Verification items for the finished model (mm, model axes). Face numbers are marked on the shaded views. Round coordinates to 2 decimals unless told otherwise and drop trailing zeros. Loops run counter-clockwise (first coordinate to the right, second up) from the corner with the lowest first, then second, coordinate; pieces in that order, holes last. Notation, with made-up numbers: (48.5, -34) - (78.5, -34) arc R23 ccw to (78.5, -26) - close; hole circle Ø7 at (31.5, 12). An arc over 180 degrees is marked (long way). Use CSV: the item, a comma, the result in double quotes.
```python
from build123d import *

# Parameters (mm, degrees)
SKETCH1_W           = 399
SKETCH1_H           = 246
BOSS_EXTRUDE1_DEPTH = 18
SKETCH2_W           = 239
SKETCH2_H           = 86
CUT_EXTRUDE1_DEPTH  = 6
CUT_EXTRUDE2_REACH  = 290.215


with BuildPart() as part:
    # Sketch1 → Boss-Extrude1 (new body)
    with BuildSketch(Plane(origin=(0, 0, 0), x_dir=(1, 0, 0), z_dir=(0, 1, 0))):
        with Locations((26.513776337, -54.93719611)):
            Rectangle(SKETCH1_W, SKETCH1_H)
    extrude(amount=BOSS_EXTRUDE1_DEPTH)

    # Sketch2 → Cut-Extrude1 (cut)
    with BuildSketch(Plane.XZ):
        with Locations((26.513776337, 54.93719611)):
            Rectangle(SKETCH2_W, SKETCH2_H)
    extrude(amount=-CUT_EXTRUDE1_DEPTH, mode=Mode.SUBTRACT)

    # Sketch3 → Cut-Extrude2 (cut, up to next)
    with BuildSketch(Plane(origin=(0, 18, 0), x_dir=(1, 0, 0), z_dir=(0, 1, 0)), mode=Mode.PRIVATE) as cut_extrude2_sk1:
        Polygon((34.013776337, 68.06280389), (19.013776337, 68.06280389), (11.513776337, 50.06280389), (11.513776337, 30.06280389), (41.513776337, 30.06280389), (41.513776337, 50.06280389), align=None)
    cut_extrude2_tool1 = extrude(cut_extrude2_sk1.sketch, amount=-CUT_EXTRUDE2_REACH, mode=Mode.PRIVATE) & part.part
    add(cut_extrude2_tool1.solids().sort_by_distance((26.513776, 18, -47.316535))[0], mode=Mode.SUBTRACT)


solid = part.part
```
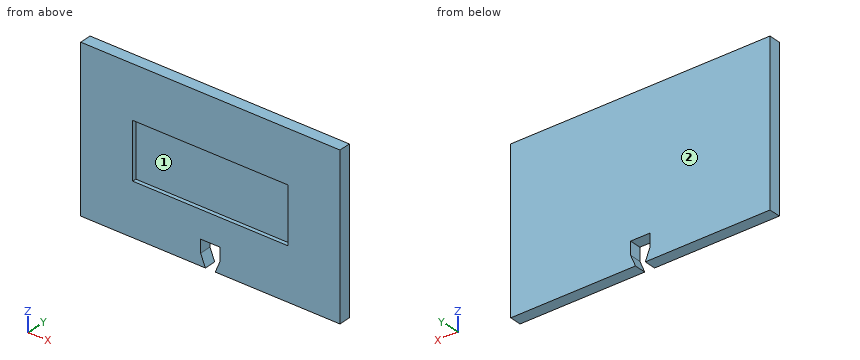
1) Cross-section at A-A, the plane y = 3. Record the cut outline in (x, z).
Returned:
outline,"(-172.99, -68.06) - (19.01, -68.06) - (11.51, -50.06) - (11.51, -30.06) - (41.51, -30.06) - (41.51, -50.06) - (34.01, -68.06) - (226.01, -68.06) - (226.01, 177.94) - (-172.99, 177.94) - close; hole (-92.99, 11.94) - (146.01, 11.94) - (146.01, 97.94) - (-92.99, 97.94) - close"
2) Thickness scan on probe 1 along Z at (x, y) = (30, 13.75); probe 2 along X at (y, z) = (5.5, 16); probe 3 along X at (y, z) = (11.5, -46). Record the ranges inside material, lowest first. Write a range as [from, to].
Returned:
probe 1,"z = [-30.06, 177.94]"
probe 2,"x = [-172.99, -92.99], [146.01, 226.01]"
probe 3,"x = [-172.99, 11.51], [41.51, 226.01]"
3) Cross-section at C-C, the plane x = 119. Record the cut outline in (y, z), then the cut area to 3 significant figures.
Returned:
outline,"(0, -68.06) - (18, -68.06) - (18, 177.94) - (0, 177.94) - (0, 97.94) - (6, 97.94) - (6, 11.94) - (0, 11.94) - close"
area,"3,910 mm²"
4) Cross-section at B-B, the plane z = 40.5. Record the cut outline in (x, y).
Returned:
outline,"(-172.99, 0) - (-92.99, 0) - (-92.99, 6) - (146.01, 6) - (146.01, 0) - (226.01, 0) - (226.01, 18) - (-172.99, 18) - close"
5) Gauge pin test, flat end, axial feed: pin 1 Ø1 at (x, z) = (64.5, 18) entering from -Y. Record the tip position at first contact, or that the pin passes through.
Returned:
pin 1,"stops at y = 6"
6) Mould release check, pull along Z, two halves, no side actions. Record for the marked faces 1 and 2: +Z half, -Z half, draft (parallel to the pull), parting line (faces both ways), or undercut.
Returned:
face 1,"undercut"
face 2,"draft"
